```python
from build123d import *

# Parameters (mm, degrees)
F2_R     = 38.1
F2_R_2   = 20.6502
F3_DEPTH = 44.45
F5_D     = 8.255


with BuildPart() as f1:
    # F0 (on Front) → F1 (revolve)
    with BuildSketch(Plane.XZ):
        Polygon((0, 50.8), (0, 17.4625), (48.26, 17.4625), (48.26, 41.275), (31.75, 41.275), (31.75, 63.5), (25.4, 52.07), align=None)
    revolve(axis=Axis((41.694678, 0, 0), (1, 0, 0)))

    # F2 (on face) → F3 (cut)
    with BuildSketch(Plane.YZ.offset(48.26)):
        Circle(F2_R)
        Circle(F2_R_2, mode=Mode.SUBTRACT)
    extrude(amount=-F3_DEPTH, mode=Mode.SUBTRACT)

    # F5 (through all)
    with Locations(Plane(origin=(0, 0, 0), x_dir=(0, 1, 0), z_dir=(-1, 0, 0))):
        with Locations((-34.925, 0), (0, -34.925), (34.925, 0), (0, 34.925)):
            Hole(F5_D / 2)


solid = f1.part
```
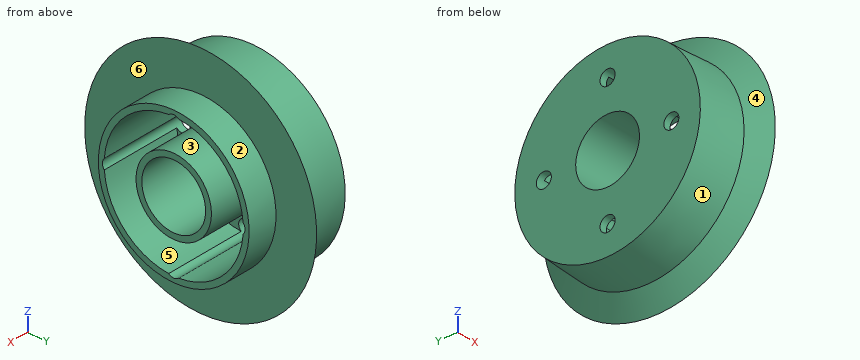
Could you check a few things on this model? Use its own coordinates, in mm. Face numbers are marked on the shaded views. A direction names the side the tool comes from. Round coordinates to 2 decimals unless told otherwise and drop trailing zeros. Answer as CSV lines item,"result".
1) For pin 1 Ø7.5 at (y, z) = (0, 34.925) entering from -X; pin 2 Ø2 at (x, y) = (25.5, -17.5) entering from +Z; pin 3 Ø12 at (x, y) = (26.5, -45) entering from +Z; pin 4 Ø5 at (x, y) = (23.5, -12) entering from +Z, each with a flat end and sliding along its axis, tell me the tip position at first contact or that it passes through.
From the geometry:
pin 1,"through"
pin 2,"z = 51.17"
pin 3,"z = 47.54"
pin 4,"z = 51.81"
2) If I drill on probe 1 along Z at (x, y) = (32, 0) (1 decimal); probe 2 along Z at (x, y) = (18.5, 16); probe 3 along Z at (x, y) = (12.5, -18.5) (3 decimals), over which ranges is the centre line in solid material (lowest first)?
From the geometry:
probe 1,"-41.3 to -39.1, -20.7 to -17.5, 17.5 to 20.7, 39.1 to 41.3"
probe 2,"-49.19 to -34.58, -13.05 to -7, 7 to 13.05, 34.58 to 49.19"
probe 3,"-47.982 to -33.307, -9.175 to 9.175, 33.307 to 47.982"
3) Which directions (+Z, -Z, +X, -X, +Y, -Y) give clear straight access to the entire face, cutting with the end or side of a thin tool? Please do the marked faces 1 and 2.
From the geometry:
face 1,"-X"
face 2,"+X"
4) Imagine slicing it at A-A on x = 35. Count the separate pieces of the cut face and the enclosed holes in it, and give its area (3 significant figures).
From the geometry:
separate pieces,"2"
enclosed holes,"2"
area,"1,160 mm^2"
5) We'd pull the mould along Z, two halves only. Please class the marked faces 3, 4, 5 and 6: released by +Z, released by -Z, zero draft, split by the parting line, or undercut.
From the geometry:
face 3,"undercut"
face 4,"split by the parting line"
face 5,"undercut"
face 6,"zero draft"
